from build123d import *

# Parameters (mm, degrees)
EXTRUDE_1_DEPTH     = 35
CUT_EXTRUDE_1_REACH = 57.803
SKETCH_2_R          = 2.2
SKETCH_3_R          = 1.7
CUT_EXTRUDE_2_DEPTH = 58.253820833


with BuildPart() as part:
    # 草图1 → 凸台-拉伸1 (new body)
    with BuildSketch(Plane.XY):
        Polygon((0, 0), (0, 42), (2, 42), (2, 2), (17, 2), (17, 0), align=None)
    extrude(amount=EXTRUDE_1_DEPTH)

    # 草图2 → 切除-拉伸1 (cut, up to next)
    with BuildSketch(Plane(origin=(0, 2, 0), x_dir=(1, 0, 0), z_dir=(0, 1, 0)), mode=Mode.PRIVATE) as cut_extrude_1_sk1:
        with Locations(Location((8, -9.5, 0), (0, 0, 180))):
            Circle(SKETCH_2_R)
    cut_extrude_1_tool1 = extrude(cut_extrude_1_sk1.sketch, amount=-CUT_EXTRUDE_1_REACH, mode=Mode.PRIVATE) & part.part
    # 草图2 → 切除-拉伸1 (cut, up to next)
    with BuildSketch(Plane(origin=(0, 2, 0), x_dir=(1, 0, 0), z_dir=(0, 1, 0)), mode=Mode.PRIVATE) as cut_extrude_1_sk2:
        with Locations(Location((8, -25.5, 0), (0, 0, 180))):
            Circle(SKETCH_2_R)
    cut_extrude_1_tool2 = extrude(cut_extrude_1_sk2.sketch, amount=-CUT_EXTRUDE_1_REACH, mode=Mode.PRIVATE) & part.part
    add(cut_extrude_1_tool1.solids().sort_by_distance((8, 2, 9.5))[0], mode=Mode.SUBTRACT)
    add(cut_extrude_1_tool2.solids().sort_by_distance((8, 2, 25.5))[0], mode=Mode.SUBTRACT)

    # 草图3 → 切除-拉伸2 (cut, through all)
    with BuildSketch(Plane.ZY):
        with Locations(Location((11.5, 10, 0), (0, 0, 270))):
            Circle(SKETCH_3_R)
        with Locations(Location((23.5, 10, 0), (0, 0, 270))):
            Circle(SKETCH_3_R)
    extrude(amount=-CUT_EXTRUDE_2_DEPTH, mode=Mode.SUBTRACT)


solid = part.part
Model file for the job. Use its own axes, mm. A direction names the side the tool comes from. Give positions to 0.01 mm unless a question says otherwise; leave off trailing zeros. Loops run counter-clockwise (first coordinate to the right, second up) from the corner with the lowest first, then second, coordinate; pieces in that order, holes last. Notation, with made-up numbers: (2.5, 14) -> (10.5, 14) arc R25 cw to (10.5, 43) -> close; hole circle Ø9 at (60, 66.25). An arc over 180 degrees is marked (long way). Use a Markdown table: item, result. Add a question column.
(1) Mould opens along Z. For faces 3 (the cylindrical face through (5.9, 1.01, 10.16)), 4 (the flat face through (1.6, 14.9, 35)), 5 (the flat face through (9, 2, 17)) say: +Z half, -Z half, draft (parallel to the pull), parting line (faces both ways), or undercut.
(2) Wall check: line 1 along Z through (x, y) = (0.7, 10); line 2 along X through (y, z) = (18, 10.5). Give the ranges that are in metal, low to high.
(3) Slice it at B-B on z = 11. List the corners of the cut face in (x, y).
(4) Drop flat-ended pins along their axis: pin 1 Ø10.5 at (y, z) = (22, 12) entering from +X; pin 2 Ø5 at (x, z) = (11.5, 24.5) entering from +Y; pin 3 Ø2.5 at (x, z) = (8, 9.5) entering from +Y. Give the stop position or say it passes through.
(5) Tool access for faces 1 (the flat face through (9, 0, 17)), 2 (the flat face through (2, 22, 17)): list every direction of +Z, -Z, +X, -X, +Y, -Y with a clear straight run to the whole face (end or side of a thin tool).
(6) Slice it at D-D on y = 13.5. List the corners of the cut face in (x, z).
(7) Slice it at C-C on z = 3. List the corners of the cut face in (x, y), and give its area (3 significant figures).
(8) Slice it at A-A on x = 8. List the corners of the cut face in (y, z).
Filled sheet:
| question | item | result |
|---|---|---|
| 1 | face 3 | undercut |
| 1 | face 4 | +Z half |
| 1 | face 5 | draft |
| 2 | line 1 | 0 to 9.8, 13.2 to 21.8, 25.2 to 35 |
| 2 | line 2 | 0 to 2 |
| 3 | outline | (0, 0) -> (6.39, 0) -> (6.39, 2) -> (2, 2) -> (2, 8.38) -> (0, 8.38) -> close; (0, 11.62) -> (2, 11.62) -> (2, 42) -> (0, 42) -> close; (9.61, 0) -> (17, 0) -> (17, 2) -> (9.61, 2) -> close |
| 4 | pin 1 | x = 2 |
| 4 | pin 2 | y = 2 |
| 4 | pin 3 | through |
| 5 | face 1 | +Z, -Z, +X, -X, -Y |
| 5 | face 2 | +Z, -Z, +X, +Y |
| 6 | outline | (0, 0) -> (2, 0) -> (2, 35) -> (0, 35) -> close |
| 7 | outline | (0, 0) -> (17, 0) -> (17, 2) -> (2, 2) -> (2, 42) -> (0, 42) -> close |
| 7 | area | 114 mm2 |
| 8 | outline | (0, 0) -> (2, 0) -> (2, 7.3) -> (0, 7.3) -> close; (0, 11.7) -> (2, 11.7) -> (2, 23.3) -> (0, 23.3) -> close; (0, 27.7) -> (2, 27.7) -> (2, 35) -> (0, 35) -> close |
